Verification items for the finished model (mm, model axes). Round coordinates to 2 decimals unless told otherwise and drop trailing zeros. Write each loop counter-clockwise with the first axis right and the second up, starting at its lowest first coordinate (ties: lowest second). Pieces come first, ordered by that corner, then holes.
from build123d import *

# Parameters (mm, degrees)
F0_W     = 92
F0_H     = 92
F0_R     = 2.25
F1_DEPTH = 3
F2_R     = 1


with BuildPart() as f1:
    # F0 (on Top) → F1 (new body)
    with BuildSketch(Plane.XY):
        Rectangle(F0_W, F0_H)
        with Locations((-41.25, -41.25)):
            Circle(F0_R, mode=Mode.SUBTRACT)
        with BuildLine():
            ThreePointArc((-6.933505, -17.526739), (-16.323145, -9.424172), (-18.645354, 2.758778))
            ThreePointArc((-18.645354, 2.758778), (-16.0832, 2.660706), (-13.58927, 2.065258))
            ThreePointArc((-13.58927, 2.065258), (-11.903787, -6.872655), (-5.006069, -12.801282))
            ThreePointArc((-5.006069, -12.801282), (-5.737361, -15.258813), (-6.933505, -17.526739))
        make_face(mode=Mode.SUBTRACT)
        with BuildLine():
            ThreePointArc((-32.485448, -21.064883), (-32.155826, -21.524565), (-31.815096, -21.976076))
            ThreePointArc((-31.815096, -21.976076), (-16.852854, -30.72923), (0, -26.671184))
            ThreePointArc((0, -26.671184), (17.411393, -30.639834), (32.485448, -21.064883))
            Line((32.485448, -21.064883), (41, -25.980762))
            Line((41, -25.980762), (41, -37.007359))
            ThreePointArc((41, -37.007359), (38.244796, -38.244796), (37.007359, -41))
            Line((37.007359, -41), (-37.007359, -41))
            ThreePointArc((-37.007359, -41), (-38.244796, -38.244796), (-41, -37.007359))
            Line((-41, -37.007359), (-41, -25.980762))
            Line((-41, -25.980762), (-32.485448, -21.064883))
        make_face(mode=Mode.SUBTRACT)
        with BuildLine():
            ThreePointArc((39.013932, -41), (41.375194, -39.003486), (43.5, -41.25))
            ThreePointArc((43.5, -41.25), (41.124806, -43.496514), (39.013932, -41))
        make_face(mode=Mode.SUBTRACT)
        with BuildLine():
            Line((3.106614, -2.604224), (5.139537, -3.777932))
            ThreePointArc((5.139537, -3.777932), (9.820807, -22.141646), (28.619151, -19.741116))
            Line((28.619151, -19.741116), (29.838639, -20.445188))
            ThreePointArc((29.838639, -20.445188), (15.574425, -28.370131), (0, -23.500859))
            ThreePointArc((0, -23.500859), (-15.573952, -28.370179), (-29.838057, -20.44594))
            Line((-29.838057, -20.44594), (-28.618517, -19.741839))
            ThreePointArc((-28.618517, -19.741839), (-9.821108, -22.141851), (-5.138765, -3.779435))
            Line((-5.138765, -3.779435), (-3.105514, -2.605536))
            ThreePointArc((-3.105514, -2.605536), (0.000856, -4.053768), (3.106614, -2.604224))
        make_face(mode=Mode.SUBTRACT)
        with BuildLine():
            ThreePointArc((18.645354, 2.758778), (16.323145, -9.424172), (6.933505, -17.526739))
            ThreePointArc((6.933505, -17.526739), (5.737361, -15.258813), (5.006069, -12.801282))
            ThreePointArc((5.006069, -12.801282), (11.903787, -6.872655), (13.58927, 2.065258))
            ThreePointArc((13.58927, 2.065258), (16.0832, 2.660706), (18.645354, 2.758778))
        make_face(mode=Mode.SUBTRACT)
        with BuildLine():
            Line((-41, -21.36196), (-41, 37.007359))
            ThreePointArc((-41, 37.007359), (-38.244796, 38.244796), (-37.007359, 41))
            Line((-37.007359, 41), (-2, 41))
            Line((-2, 41), (-2, 38.665665))
            ThreePointArc((-2, 38.665665), (-2.562907, 38.610045), (-3.124292, 38.54072))
            ThreePointArc((-3.124292, 38.54072), (-18.185867, 29.959614), (-23.097923, 13.335592))
            ThreePointArc((-23.097923, 13.335592), (-35.240571, 0.241208), (-34.485448, -17.600782))
            Line((-34.485448, -17.600782), (-41, -21.36196))
        make_face(mode=Mode.SUBTRACT)
        with BuildLine():
            Line((-0.703704, 6.340019), (-0.703704, 3.992222))
            ThreePointArc((-0.703704, 3.992222), (-3.511094, 2.026142), (-3.808631, -1.388295))
            Line((-3.808631, -1.388295), (-5.841554, -2.562003))
            ThreePointArc((-5.841554, -2.562003), (-24.085631, 2.565755), (-31.405884, -14.914353))
            Line((-31.405884, -14.914353), (-32.625372, -15.618425))
            ThreePointArc((-32.625372, -15.618425), (-32.356466, 0.697218), (-20.352341, 11.75043))
            ThreePointArc((-20.352341, 11.75043), (-16.78232, 27.672527), (-2.787675, 36.063485))
            Line((-2.787675, 36.063485), (-2.787675, 34.655283))
            ThreePointArc((-2.787675, 34.655283), (-14.264851, 19.576254), (-0.703704, 6.340019))
        make_face(mode=Mode.SUBTRACT)
        with BuildLine():
            ThreePointArc((-41, 39.013932), (-42.927051, 42.75), (-39, 41.25))
            ThreePointArc((-39, 41.25), (-39.572949, 39.75), (-41, 39.013932))
        make_face(mode=Mode.SUBTRACT)
        with BuildLine():
            Line((0.702017, 3.992519), (0.702017, 6.339936))
            ThreePointArc((0.702017, 6.339936), (14.264824, 19.575891), (2.786733, 34.65547))
            Line((2.786733, 34.65547), (2.786733, 36.063613))
            ThreePointArc((2.786733, 36.063613), (16.782041, 27.672913), (20.352341, 11.75043))
            ThreePointArc((20.352341, 11.75043), (32.356272, 0.697652), (32.625732, -15.617545))
            Line((32.625732, -15.617545), (31.406193, -14.913444))
            ThreePointArc((31.406193, -14.913444), (24.085959, 2.565596), (5.842469, -2.560584))
            Line((5.842469, -2.560584), (3.809217, -1.386686))
            ThreePointArc((3.809217, -1.386686), (3.510238, 2.027625), (0.702017, 3.992519))
        make_face(mode=Mode.SUBTRACT)
        with BuildLine():
            ThreePointArc((34.485448, -17.600782), (34.718733, -17.08548), (34.939388, -16.564644))
            ThreePointArc((34.939388, -16.564644), (35.03872, 0.769615), (23.097923, 13.335592))
            ThreePointArc((23.097923, 13.335592), (17.829178, 30.398626), (2, 38.665665))
            Line((2, 38.665665), (2, 41))
            Line((2, 41), (37.007359, 41))
            ThreePointArc((37.007359, 41), (38.244796, 38.244796), (41, 37.007359))
            Line((41, 37.007359), (41, -21.36196))
            Line((41, -21.36196), (34.485448, -17.600782))
        make_face(mode=Mode.SUBTRACT)
        with BuildLine():
            ThreePointArc((-11.711849, 14.767961), (0, 18.848344), (11.711849, 14.767961))
            ThreePointArc((11.711849, 14.767961), (10.345839, 12.598107), (8.583201, 10.736024))
            ThreePointArc((8.583201, 10.736024), (0, 13.74531), (-8.583201, 10.736024))
            ThreePointArc((-8.583201, 10.736024), (-10.345839, 12.598107), (-11.711849, 14.767961))
        make_face(mode=Mode.SUBTRACT)
        with Locations((41.25, 41.25)):
            Circle(F0_R, mode=Mode.SUBTRACT)
    extrude(amount=F1_DEPTH)

    # F2
    f2_edges = [f1.edges().sort_by_distance(p)[0] for p in [
        (0, 46, 3),
        (46, 0, 3),
        (-46, 0, 3),
        (0, -46, 3),
    ]]
    fillet(f2_edges, radius=F2_R)


solid = f1.part
Q1. Material ranges on line 1 along Y through (x, z) = (-41.25, 1.25); line 2 along X through (y, z) = (40.5, 2.45); line 3 along X through (y, z) = (-26, 2.7), recorded low to high.
Recorded:
line 1: y = -46 to -43.5, -39 to 39, 43.5 to 46
line 2: x = -45.89 to -43.37, -39.13 to -37.07, -2 to 2, 37.07 to 39.13, 43.37 to 45.89
line 3: x = -45.71 to -41, -27.83 to -23.29, -3.64 to 3.64, 23.29 to 27.83, 41 to 45.71
Q2. Sectioned sample at D-D (x = 27). Enter the section's corners in (y, z).
Recorded:
outline: (-46, 0) - (-41, 0) - (-41, 3) - (-45, 3) arc R1 ccw to (-46, 2) - close; (-26.62, 0) - (-23.44, 0) - (-23.44, 3) - (-26.62, 3) - close; (-21.32, 0) - (0.69, 0) - (0.69, 3) - (-21.32, 3) - close; (7.89, 0) - (11.07, 0) - (11.07, 3) - (7.89, 3) - close; (41, 0) - (46, 0) - (46, 2) arc R1 ccw to (45, 3) - (41, 3) - close
Q3. Release check for a two-part mould opening along X. For faces 1 (the flat face through (2, 40, 1)), 2 (the cylindrical face through (-32.451, 0.482, 1.479)) record: released by +X, released by -X, zero draft, split by the parting line, or undercut.
Recorded:
face 1: undercut
face 2: undercut
Q4. Sectioned sample at B-B (x = 16). Enter the section's corners in (y, z), plus the area to 3 significant figures.
Recorded:
outline: (-46, 0) - (-41, 0) - (-41, 3) - (-45, 3) arc R1 ccw to (-46, 2) - close; (-30.84, 0) - (-28.32, 0) - (-28.32, 3) - (-30.84, 3) - close; (-24.49, 0) - (-9.96, 0) - (-9.96, 3) - (-24.49, 3) - close; (2.65, 0) - (3.87, 0) - (3.87, 3) - (2.65, 3) - close; (28.69, 0) - (32.35, 0) - (32.35, 3) - (28.69, 3) - close; (41, 0) - (46, 0) - (46, 2) arc R1 ccw to (45, 3) - (41, 3) - close
area: 95.4 mm2
Q5. Depth check by flat-ended pin: P1, Ø1, axis at x = -35.5, y = -20, coming from the -Z side; P2, Ø3.5, axis at x = 41.25, y = 41.25, coming from the +Z side. Enter the tip coordinate at first touch or a pass-through.
Recorded:
P1: stops at z = 0
P2: passes through
Q6. Sectioned sample at C-C (y = -9). Give the number of separate pieces and of enclosed holes in the cut face, plus the area to 3 significant figures.
Recorded:
separate pieces: 8
enclosed holes: 0
area: 178 mm2
Q7. Sectioned sample at A-A (y = -34.5). Enter the section's corners in (x, z).
Recorded:
outline: (-46, 0) - (-41, 0) - (-41, 3) - (-45, 3) arc R1 ccw to (-46, 2) - close; (41, 0) - (46, 0) - (46, 2) arc R1 ccw to (45, 3) - (41, 3) - close
